```python
from build123d import *

# Parameters (mm, degrees)
MODEL_R                  = 7.35
MODEL_R_2                = 7.3
MODEL_R_3                = 1.85
RESSALTO_EXTRUS_O1_DEPTH = 8
ESBO_O3_R                = 11.3
CORTE_EXTRUS_O1_DEPTH    = 2
ESBO_O4_R                = 11.3
CORTE_EXTRUS_O2_DEPTH    = 2
ESBO_O2_R                = 3.3
CORTE_EXTRUS_O4_DEPTH    = 2
ESBO_O6_R                = 1.5
CORTE_EXTRUS_O5_DEPTH    = 10
ESBO_O7_R                = 1.5
SUPOERTE_PLACA_DEPTH     = 9


with BuildPart() as part:
    # Model → Ressalto-extrusão1 (new body)
    with BuildSketch(Plane.XY):
        with BuildLine():
            Line((0, 0), (39, 0))
            Line((39, 0), (39.7, 0))
            Line((39.7, 0), (39.7, -6.854833996))
            Line((39.7, -6.854833996), (52.445166004, -19.6))
            Line((52.445166004, -19.6), (59.445166004, -26.6))
            Line((59.445166004, -26.6), (81.699998871, -26.6))
            ThreePointArc((81.699998871, -26.6), (102.949229032, -12.401719466), (97.963455967, 12.663455967))
            Line((97.963455967, 12.663455967), (63.677897161, 46.949014774))
            Line((63.677897161, 46.949014774), (50.111140335, 46.949014774))
            Line((50.111140335, 46.949014774), (15.50707852, 46.949014774))
            Line((15.50707852, 46.949014774), (0, 31.441936254))
            Line((0, 31.441936254), (0, 0))
        make_face()
        with Locations((59.072583002, 19.027416998)):
            Circle(MODEL_R, mode=Mode.SUBTRACT)
        with Locations((81.7, -3.6)):
            Circle(MODEL_R_2, mode=Mode.SUBTRACT)
        with Locations((6.960594046, 15.730973227)):
            Circle(MODEL_R_3, mode=Mode.SUBTRACT)
        with Locations((6.960594046, 31.230973227)):
            Circle(MODEL_R_3, mode=Mode.SUBTRACT)
        with Locations((20.383987804, 38.980973227)):
            Circle(MODEL_R_3, mode=Mode.SUBTRACT)
        with Locations((33.807381563, 31.230973227)):
            Circle(MODEL_R_3, mode=Mode.SUBTRACT)
        with Locations((33.807381563, 15.730973227)):
            Circle(MODEL_R_3, mode=Mode.SUBTRACT)
        with Locations((20.383987804, 7.980973227)):
            Circle(MODEL_R_3, mode=Mode.SUBTRACT)
        with Locations((27.383987804, 23.480973227)):
            Circle(MODEL_R, mode=Mode.SUBTRACT)
        Polygon((72, -15), (52, 5), (45, 5), (45, -4), (61, -20), (77, -20), align=None, mode=Mode.SUBTRACT)
    extrude(amount=RESSALTO_EXTRUS_O1_DEPTH)

    # Esboço3 → Corte-extrusão1 (cut)
    with BuildSketch(Plane.XY):
        with Locations((81.7, -3.6)):
            Circle(ESBO_O3_R)
        with Locations((59.0726, 19.0274)):
            Circle(ESBO_O3_R)
        with Locations((27.384004802, 23.480956229)):
            Circle(ESBO_O3_R)
    extrude(amount=CORTE_EXTRUS_O1_DEPTH, mode=Mode.SUBTRACT)

    # Esboço4 → Corte-extrusão2 (cut)
    with BuildSketch(Plane.XY.offset(8)):
        with Locations((81.7, -3.6)):
            Circle(ESBO_O4_R)
        with Locations((59.0726, 19.0274)):
            Circle(ESBO_O4_R)
        with Locations((27.384004802, 23.480956229)):
            Circle(ESBO_O4_R)
    extrude(amount=-CORTE_EXTRUS_O2_DEPTH, mode=Mode.SUBTRACT)

    # Esboço2 → Corte-extrusão4 (cut)
    with BuildSketch(Plane.XY):
        with Locations((6.960594802, 15.730956229)):
            Circle(ESBO_O2_R)
        with Locations((6.960594802, 31.230956229)):
            Circle(ESBO_O2_R)
        with Locations((33.807404802, 15.730956229)):
            Circle(ESBO_O2_R)
        with Locations((20.384004802, 38.980956229)):
            Circle(ESBO_O2_R)
        with Locations((33.807404802, 31.230956229)):
            Circle(ESBO_O2_R)
        with Locations((20.384004802, 7.980976229)):
            Circle(ESBO_O2_R)
    extrude(amount=CORTE_EXTRUS_O4_DEPTH, mode=Mode.SUBTRACT)

    # Esboço6 → Corte-extrusão5 (cut)
    with BuildSketch(Plane.XZ):
        with Locations((11.8, 4)):
            Circle(ESBO_O6_R)
        with Locations((30.8, 4)):
            Circle(ESBO_O6_R)
    extrude(amount=-CORTE_EXTRUS_O5_DEPTH, mode=Mode.SUBTRACT)

    # Esboço7 → supoerte_placa (cut, through all)
    with BuildSketch(Plane.XY.offset(8)):
        with Locations((27.383987804, 38.980973227)):
            Circle(ESBO_O7_R)
        with Locations((41.383987804, 38.980973227)):
            Circle(ESBO_O7_R)
        with Locations((41.383987804, 7.980973227)):
            Circle(ESBO_O7_R)
        with Locations((27.383987804, 7.980973227)):
            Circle(ESBO_O7_R)
    extrude(amount=-SUPOERTE_PLACA_DEPTH, mode=Mode.SUBTRACT)


solid = part.part
```
Source: CAD feature listing. Evaluate the final solid. Frame: model axes, mm. A direction names the side the tool comes from. Round coordinates to 2 decimals unless told otherwise and drop trailing zeros. Loops run counter-clockwise (first coordinate to the right, second up) from the corner with the lowest first, then second, coordinate; pieces in that order, holes last.
1. Contact query for flat-ended pins moving along their axis: pin 1 (2 mm diameter, centred on y = -7, z = 6.5, fed in from +X); pin 2 (18 mm diameter, centred on x = 27.38, y = 23.48, fed in from +Z); pin 3 (2 mm diameter, centred on x = 20.38, y = 38.98, fed in from -Z) (3 decimals); pin 4 (1 mm diameter, centred on y = -16, z = 4, fed in from -X). Output: stop coordinate, or through.
2. Access query for faces 4 (the flat face through (89, -6, 6)), 5 (the cylindrical face through (8.48, 28.3, 0.99)), 6 (the flat face through (49.434, -16.589, 3.944)), 7 (the flat face through (49, 5, 4)). Directions: +Z, -Z, +X, -X, +Y, -Y. A direction counts if a zero-diameter tool reaches every point of the face in a straight line with its end or side. Return the directions, or none.
3. Ray query, L1, parallel to Y at x = 59.5, z = 6.75; L2, parallel to X at y = 19.5, z = 6.5; L3, parallel to Y at x = 69.5, z = 1.25. Return the intervals inside material, ascending.
4. Section query B-B on x = 50. Output: boundary loops of the cut face in (y, z), and give its area (3 significant figures).
5. Section query D-D on x = 27.5. Output: boundary loops of the cut face in (y, z), and give its area (3 significant figures).
6. Section query C-C on y = -13. Output: boundary loops of the cut face in (x, z).
7. Section query A-A on y = 2. Output: boundary loops of the cut face in (x, z).
8. Mould query, pull axis Y, two halves, no side actions, for faces 1 (the flat face through (12, 10, 4)), 2 (the flat face through (66.4, 16.7, 2)), 3 (the cylindrical face through (102.8, -12.75, 3.94)). Classes: released by +Y, released by -Y, zero draft, split by the parting line, or undercut.
Answers below:
1. pin 1: stops at x = 104.57
1. pin 2: stops at z = 6
1. pin 3: passes through
1. pin 4: stops at x = 48.35
2. face 4: +Z
2. face 5: -Z
2. face 6: +Z, -Z, -X, -Y
2. face 7: +Z, -Z
3. L1: y = -26.6 to -18.5, -2.5 to 7.74, 30.32 to 46.95
3. L2: x = 0 to 16.81, 37.96 to 47.78, 70.36 to 91.13
3. L3: y = -26.6 to -20, -12.5 to 14.67, 23.38 to 41.13
4. outline: (-17.15, 0) - (-9, 0) - (-9, 8) - (-17.15, 8) - close; (5, 0) - (12.29, 0) - (12.29, 2) - (25.76, 2) - (25.76, 0) - (46.95, 0) - (46.95, 8) - (25.76, 8) - (25.76, 6) - (12.29, 6) - (12.29, 8) - (5, 8) - close
4. area: 347 mm2
5. outline: (0, 0) - (6.49, 0) - (6.49, 8) - (0, 8) - close; (9.48, 0) - (12.18, 0) - (12.18, 2) - (16.13, 2) - (16.13, 6) - (12.18, 6) - (12.18, 8) - (9.48, 8) - close; (30.83, 2) - (34.78, 2) - (34.78, 0) - (37.49, 0) - (37.49, 8) - (34.78, 8) - (34.78, 6) - (30.83, 6) - close; (40.48, 0) - (46.95, 0) - (46.95, 8) - (40.48, 8) - close
5. area: 179 mm2
6. outline: (45.85, 0) - (54, 0) - (54, 8) - (45.85, 8) - close; (70, 0) - (75.43, 0) - (75.43, 2) - (87.97, 2) - (87.97, 0) - (102.69, 0) - (102.69, 8) - (87.97, 8) - (87.97, 6) - (75.43, 6) - (75.43, 8) - (70, 8) - close
7. outline: (0, 0) - (45, 0) - (45, 8) - (0, 8) - close; (55, 0) - (71.89, 0) - (71.89, 2) - (77.02, 2) - (77.02, 6) - (71.89, 6) - (71.89, 8) - (55, 8) - close; (86.38, 2) - (91.51, 2) - (91.51, 0) - (104.01, 0) - (104.01, 8) - (91.51, 8) - (91.51, 6) - (86.38, 6) - close; hole circle Ø3 at (11.8, 4); hole circle Ø3 at (30.8, 4)
8. face 1: released by -Y
8. face 2: undercut
8. face 3: split by the parting line
